Geometry check sheet. Reference: the model listing, model coordinates, mm. Face numbers are marked on the shaded views. A direction names the side the tool comes from. Round coordinates to 2 decimals unless told otherwise and drop trailing zeros. Loops run counter-clockwise (first coordinate to the right, second up) from the corner with the lowest first, then second, coordinate; pieces in that order, holes last. Notation, with made-up numbers: (-6, -17) - (39, -17) arc R32 ccw to (39, 11) - close; hole circle Ø4 at (9, -19). An arc over 180 degrees is marked (long way). Answer as CSV lines item,"result". Start each with the question number.
1) Depth check by flat-ended pin: P1, Ø5, axis at y = 1, z = -22.5, coming from the +X side; P2, Ø2, axis at y = 18, z = -19, coming from the +X side; P3, Ø8, axis at x = -7.5, z = -2.5, coming from the +Y side. Enter the tip coordinate at first touch or a pass-through.
2) Cross-section at C-C on y = -13.5. Record the boundary of the cut face in (x, z).
3) Cross-section at B-B on x = 0. Record the boundary of the cut face in (y, z), and give its area (3 significant figures).
4) Access from +Z, -Z, +X, -X, +Y, -Y to the whole of each face (thin tool, end or side, straight path). Record for the marked faces 5, 6 and 7.
5) Cross-section at A-A on z = 0. Record the boundary of the cut face in (x, y), and give its area (3 significant figures).
6) Thickness scan on line 1 along Z through (x, y) = (0, -17); line 2 along Y through (x, z) = (6.5, 14); line 3 along Z through (x, y) = (-4.5, -15.5). Record the ranges inside material, lowest first.
7) Draft check along X on the marked faces 1, 2, 3 and 4. Enter one of: released by +X, released by -X, zero draft, split by the parting line, or undercut.
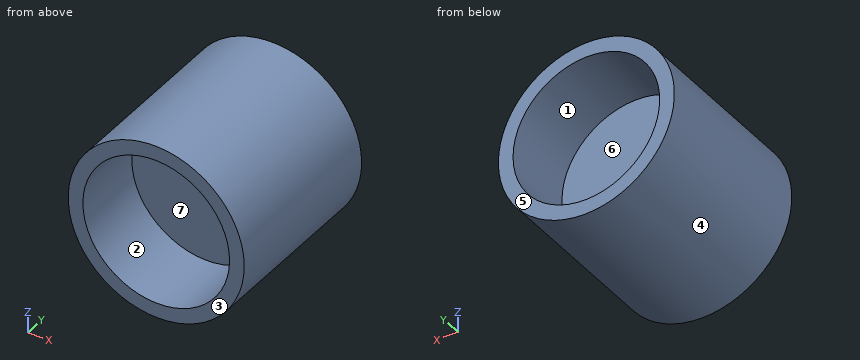
from build123d import *

# Parameters (mm, degrees)
F0_R     = 30
F1_DEPTH = 30
F2_R     = 25
F3_DEPTH = 25


with BuildPart() as f1:
    # F0 (on Front) → F1 (new body)
    with BuildSketch(Plane.XZ):
        Circle(F0_R)
    extrude(amount=F1_DEPTH)

    # F2 (on face) → F3 (cut)
    with BuildSketch(Plane.XZ.offset(30)):
        Circle(F2_R)
    extrude(amount=-F3_DEPTH, mode=Mode.SUBTRACT)

    # F4: F1 across plane


with BuildPart() as f1_1:
    add(f1.part)
    add(f1.part.mirror(Plane.XZ))


solid = f1_1.part
Answer block:
1,P1,"stops at x = 22.36"
1,P2,"stops at x = 24"
1,P3,"stops at y = 5"
2,outline,"circle Ø60 at (0, 0); hole circle Ø50 at (0, 0)"
3,outline,"(-30, -30) - (30, -30) - (30, -25) - (5, -25) - (5, 25) - (30, 25) - (30, 30) - (-30, 30) - (-30, 25) - (-5, 25) - (-5, -25) - (-30, -25) - close"
3,area,"1,100 mm^2"
4,face 5,"+Z, -Z, +X, -X, +Y"
4,face 6,"+Y"
4,face 7,"-Y"
5,outline,"(-30, -30) - (-25, -30) - (-25, -5) - (25, -5) - (25, -30) - (30, -30) - (30, 30) - (25, 30) - (25, 5) - (-25, 5) - (-25, 30) - (-30, 30) - close"
5,area,"1,100 mm^2"
6,line 1,"z = -30 to -25, 25 to 30"
6,line 2,"y = -5 to 5"
6,line 3,"z = -29.66 to -24.59, 24.59 to 29.66"
7,face 1,"undercut"
7,face 2,"undercut"
7,face 3,"zero draft"
7,face 4,"split by the parting line"
